Build history of the part. All positions in model axes, mm. Face numbers are marked on the shaded views. Give positions to 0.01 mm unless a question says otherwise; leave off trailing zeros. Order: outer loops, then holes, each group sorted by start corner. A loop starts at its lowest first (then second) coordinate and runs counter-clockwise, first axis right, second up. Notation, with made-up numbers: M 0.5,6 L 59.5,6 A12 ccw 59.5,18 Z; hole C 7,56.25 d10. An arc over 180 degrees is marked long. Answer as CSV lines item,"result".
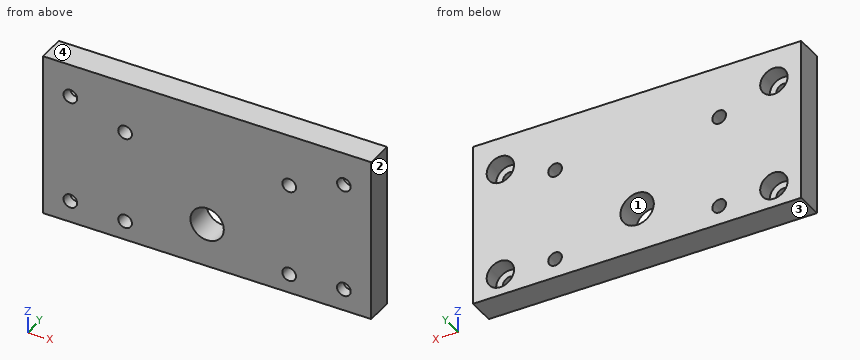
from build123d import *

# Parameters (mm, degrees)
SKETCH1_W           = 60
SKETCH1_H           = 30
BOSS_EXTRUDE1_DEPTH = 5
SKETCH2_R           = 3.05
SKETCH2_R_2         = 1.25
CUT_EXTRUDE1_DEPTH  = 5
SKETCH3_R           = 1.25
CUT_EXTRUDE2_DEPTH  = 5
SKETCH4_R           = 2.5
CUT_EXTRUDE3_DEPTH  = 3


with BuildPart() as part:
    # Sketch1 → Boss-Extrude1 (new body)
    with BuildSketch(Plane(origin=(0, 0, 0), x_dir=(1, 0, 0), z_dir=(0, 1, 0))):
        with Locations((30, 15)):
            Rectangle(SKETCH1_W, SKETCH1_H)
    extrude(amount=BOSS_EXTRUDE1_DEPTH)

    # Sketch2 → Cut-Extrude1 (cut)
    with BuildSketch(Plane(origin=(0, 5, 0), x_dir=(1, 0, 0), z_dir=(0, 1, 0))):
        with Locations((30, 22)):
            Circle(SKETCH2_R)
        with Locations((45, 26.5)):
            Circle(SKETCH2_R_2)
        with Locations((45, 9.5)):
            Circle(SKETCH2_R_2)
    cut_extrude1 = extrude(amount=-CUT_EXTRUDE1_DEPTH, mode=Mode.SUBTRACT)

    # Mirror1: Cut-Extrude1 across plane
    add(cut_extrude1.mirror(Plane.ZY.offset(-30)), mode=Mode.SUBTRACT)

    # Sketch3 → Cut-Extrude2 (cut)
    with BuildSketch(Plane(origin=(0, 5, 0), x_dir=(1, 0, 0), z_dir=(0, 1, 0))):
        with Locations((55, 26)):
            Circle(SKETCH3_R)
        with Locations((55, 6)):
            Circle(SKETCH3_R)
    cut_extrude2 = extrude(amount=-CUT_EXTRUDE2_DEPTH, mode=Mode.SUBTRACT)

    # Mirror2: Cut-Extrude2 across plane
    add(cut_extrude2.mirror(Plane.ZY.offset(-30)), mode=Mode.SUBTRACT)

    # Sketch4 → Cut-Extrude3 (cut)
    with BuildSketch(Plane(origin=(0, 5, 0), x_dir=(1, 0, 0), z_dir=(0, 1, 0))):
        with Locations((55, 26)):
            Circle(SKETCH4_R)
        with Locations((55, 6)):
            Circle(SKETCH4_R)
    cut_extrude3 = extrude(amount=-CUT_EXTRUDE3_DEPTH, mode=Mode.SUBTRACT)

    # Mirror3: Cut-Extrude3 across plane
    add(cut_extrude3.mirror(Plane.ZY.offset(-30)), mode=Mode.SUBTRACT)


solid = part.part
Item 1: Probe line 1 along Z through (x, y) = (5, 1.3); line 2 along Z through (x, y) = (15, 2.45); line 3 along X through (y, z) = (1.8, -9.5). List the from-to ranges inside material, lowest first. Write a range as from..to.
Geometry says:
line 1,"z = -30..-27.25, -24.75..-7.25, -4.75..0"
line 2,"z = -30..-27.75, -25.25..-10.75, -8.25..0"
line 3,"x = 0..13.75, 16.25..43.75, 46.25..60"
Item 2: Band-saw the part on D-D (z = -22). Give the cut face in (x, y), and give its area (4 significant figures).
Geometry says:
outline,"M 0,0 L 26.95,0 L 26.95,5 L 0,5 Z; M 33.05,0 L 60,0 L 60,5 L 33.05,5 Z"
area,"269.5 mm2"
Item 3: Drop flat-ended pins along their axis: pin 1 (6 mm diameter, centred on x = 55, z = -26, fed in from +Y); pin 2 (2 mm diameter, centred on x = 45, z = -26.5, fed in from -Y); pin 3 (2.5 mm diameter, centred on x = 5.5, z = -26, fed in from +Y). Give the stop position or say it passes through.
Geometry says:
pin 1,"stops at y = 5"
pin 2,"passes through"
pin 3,"stops at y = 2"
Item 4: Pull direction Z, two halves, no side cores. Call the marked faces 1, 2, 3 and 4: released by +Z, released by -Z, zero draft, split by the parting line, or undercut.
Geometry says:
face 1,"undercut"
face 2,"zero draft"
face 3,"released by -Z"
face 4,"released by +Z"
Item 5: Band-saw the part on C-C (z = -9.5). Give the cut face in (x, y).
Geometry says:
outline,"M 0,0 L 13.75,0 L 13.75,5 L 0,5 Z; M 16.25,0 L 43.75,0 L 43.75,5 L 16.25,5 Z; M 46.25,0 L 60,0 L 60,5 L 46.25,5 Z"
Item 6: Band-saw the part on B-B (y = 4.15). State how many separate pieces and enclosed holes the cut face has, and give its area (3 significant figures).
Geometry says:
separate pieces,"1"
enclosed holes,"9"
area,"1,670 mm2"
Item 7: Band-saw the part on A-A (x = 15). Give the cut face in (y, z).
Geometry says:
outline,"M 0,-30 L 5,-30 L 5,-27.75 L 0,-27.75 Z; M 0,-25.25 L 5,-25.25 L 5,-10.75 L 0,-10.75 Z; M 0,-8.25 L 5,-8.25 L 5,0 L 0,0 Z"
